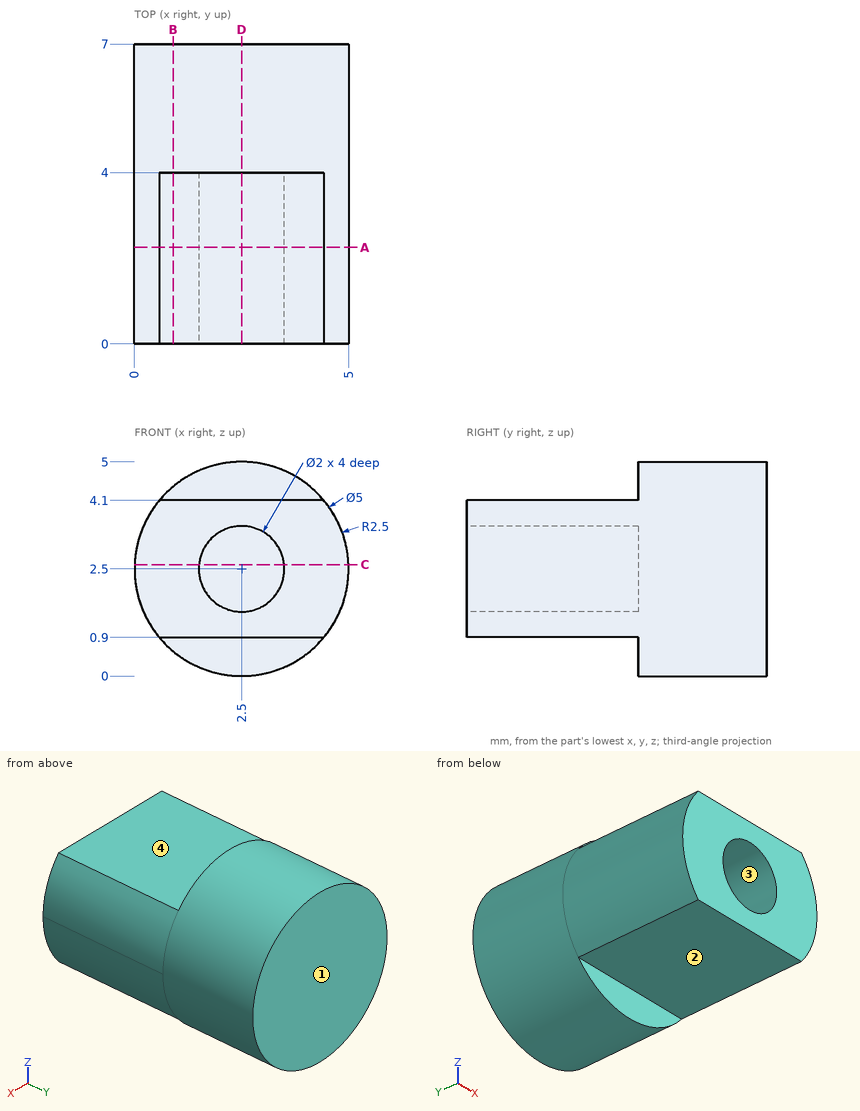
Print and shaded views of the part. All mm, measured from the part's lowest x, y and z. A direction names the side the tool comes from. Coordinates: 2 decimals unless noted, no trailing zeros. Order: outer loops, then holes, each group sorted by start corner. A loop starts at its lowest first (then second) coordinate and runs counter-clockwise, first axis right, second up. Notation, with made-up numbers: M 12.5,57 L 26.5,57 A30 ccw 26.5,80 Z; hole C 33.5,-5 d3. An arc over 180 degrees is marked long. Write each question's results on one line, items separated by ' | '. Start each with the question number.
Q1. Flat gauge pins, fed straight in: P1, Ø3, axis at y = 2.5, z = 1, coming from the -X side; P2, Ø3, axis at y = 4, z = 4.5, coming from the -X side; P3, Ø3, axis at x = 2.5, y = 1.5, coming from the -Z side; P4, Ø1.2, axis at x = 2, y = 3, coming from the +Z side. Where does each tip first touch, or does it go through?
Q2. Cut at C-C (z = 2.6). List the corners of the cut face in (x, y).
Q3. Cut at B-B (x = 0.9). List the corners of the cut face in (y, z), then the cut area to 3 significant figures.
Q4. Cut at D-D (x = 2.5). List the corners of the cut face in (y, z), then the cut area to 3 significant figures.
Q5. Which spindle directions (+Z, -Z, +X, -X, +Y, -Y) get a long thin tool onto all of the face, cutting with end or side? Do the marked faces 1 and 2. Say none if no direction does.
Q6. Pull direction X, two halves, no side cores. Call the marked faces 3 and 4: +X half, -X half, draft (parallel to the pull), parting line (faces both ways), or undercut.
Q7. Drill centre lines: probe 1 along Z at (x, y) = (2.5, 1.35); probe 2 along Y at (x, z) = (3.2, 2.35); probe 3 along Z at (x, y) = (1.2, 3.5). Where is each one in solid material? Low to high. Write a range as from..to.
Q8. Cut at A-A (y = 2.25). List the corners of the cut face in (x, z), then the cut area to 3 significant figures.
Found:
1) P1: x = 0 | P2: x = 0.05 | P3: z = 0.9 | P4: z = 4.1
2) outline: M 0,0 L 1.51,0 L 1.51,4 L 3.49,4 L 3.49,0 L 5,0 L 5,7 L 0,7 Z
3) outline: M 0,0.9 L 4,0.9 L 4,0.58 L 7,0.58 L 7,4.42 L 4,4.42 L 4,4.1 L 0,4.1 Z | area: 24.3 mm²
4) outline: M 0,0.9 L 4,0.9 L 4,0 L 7,0 L 7,5 L 4,5 L 4,4.1 L 0,4.1 L 0,3.5 L 4,3.5 L 4,1.5 L 0,1.5 Z | area: 19.8 mm²
5) face 1: +Z, -Z, +X, -X, +Y | face 2: -Z, +X, -X, -Y
6) face 3: undercut | face 4: draft
7) probe 1: 0.9..1.5, 3.5..4.1 | probe 2: 4..7 | probe 3: 0.9..4.1
8) outline: M 0.58,0.9 L 4.42,0.9 A2.5 ccw 4.42,4.1 L 0.58,4.1 A2.5 ccw Z; hole C 2.5,2.5 d2 | area: 11.7 mm²
